Read the model definition and answer for the solid it produces. Units are mm, in the model's axes. A direction names the side the tool comes from. Coordinates: 2 decimals unless noted, no trailing zeros. Write each loop counter-clockwise with the first axis right and the second up, starting at its lowest first coordinate (ties: lowest second). Pieces come first, ordered by that corner, then holes. Notation, with made-up numbers: (20.5, 56) - (74.5, 56) arc R29 ccw to (74.5, 78) - close; hole circle Ø10 at (-2.75, 3). An arc over 180 degrees is marked (long way). Use a Markdown table: item, result.
from build123d import *

# Parameters (mm, degrees)
F1_DEPTH = 3.175
F2_R     = 1.27


with BuildPart() as f1:
    # F0 (on Top) → F1 (new body)
    with BuildSketch(Plane.XY):
        with BuildLine():
            Line((-21.930882, 13.368339), (-2.54, -2.842578))
            Line((-2.54, -2.842578), (-2.54, -18.3762))
            Line((-2.54, -18.3762), (-2.54, -24.069088))
            Line((-2.54, -24.069088), (2.54, -24.069088))
            Line((2.54, -24.069088), (6.35, -24.069088))
            Line((6.35, -24.069088), (6.35, -18.3762))
            Line((6.35, -18.3762), (2.54, -18.3762))
            Line((2.54, -18.3762), (2.54, -2.842578))
            Line((2.54, -2.842578), (21.930882, 13.368339))
            ThreePointArc((21.930882, 13.368339), (23.67951, 37.005537), (0, 38.032972))
            ThreePointArc((0, 38.032972), (-23.67951, 37.005537), (-21.930882, 13.368339))
        make_face()
        with BuildLine():
            Line((19.48717, 16.291415), (0, 0))
            Line((0, 0), (-19.48717, 16.291415))
            ThreePointArc((-19.48717, 16.291415), (-19.234192, 35.984614), (0, 31.75))
            ThreePointArc((0, 31.75), (19.234192, 35.984614), (19.48717, 16.291415))
        make_face(mode=Mode.SUBTRACT)
    extrude(amount=F1_DEPTH)

    # F2
    f2_edges = [f1.edges().sort_by_distance(p)[0] for p in [
        (-12.235441, 5.262881, 3.175),
        (-23.67951, 37.005537, 3.175),
        (23.67951, 37.005537, 3.175),
        (12.235441, 5.262881, 3.175),
        (-2.54, -13.455833, 3.175),
        (2.54, -10.609389, 3.175),
        (-9.743585, 8.145707, 0),
        (-19.234192, 35.984614, 3.175),
        (19.234192, 35.984614, 3.175),
        (4.445, -18.3762, 3.175),
        (6.35, -21.222644, 3.175),
        (1.905, -24.069088, 3.175),
    ]]
    fillet(f2_edges, radius=F2_R)


solid = f1.part
(1) For faces 4 (the flat face through (-9.607, 8.032, 1.583)), 5 (the flat face through (6.35, -21, 1)), 6 (the cylindrical face through (-9.71, 7.65, 2.79)), 7 (the flat face through (4, -18.376, 1)), 8 (the cylindrical face through (11.914, 5.467, 2.793)), determine the directions among +Z, -Z, +X, -X, +Y, -Y from which every point of the face is accessible in a straight line to the end or side of a thin tool.
Report:
| item | result |
|---|---|
| face 4 | +Z, -Z |
| face 5 | +Z, -Z, +X, -Y |
| face 6 | +Z |
| face 7 | +Z, -Z, +X |
| face 8 | +Z, +X |
(2) The mould has two halves that part along Y. Classify faces 1 (the cylindrical face through (9.426, 7.409, 2.793)), 2 (the cylindrical face through (23.92, 36.73, 0.94)), 3 (the flat face through (-12.4, 5.4, 0.9)): pulls with the +Y half, pulls with the -Y half, needs draft (parallel to the pull), parting line crosses it, or undercut.
Report:
| item | result |
|---|---|
| face 1 | undercut |
| face 2 | parting line crosses it |
| face 3 | pulls with the -Y half |
(3) A cutting plane is placed at B-B, the plane y = -13. Write down the section's boundary in (x, z) (3 decimals), and give its area (3 significant figures).
Report:
| item | result |
|---|---|
| outline | (-2.54, 0) - (2.54, 0) - (2.54, 1.905) arc R1.27 ccw to (1.27, 3.175) - (-1.27, 3.175) arc R1.27 ccw to (-2.54, 1.905) - close |
| area | 15.4 mm² |
(4) A cutting plane is placed at C-C, the plane y = 35. Count the separate pieces of the cut face and the enclosed holes in it, and give its area (3 significant figures).
Report:
| item | result |
|---|---|
| separate pieces | 3 |
| enclosed holes | 0 |
| area | 42.1 mm² |
(5) Straight lines are drawn through the part: L1, parallel to X at y = 36, z = 0.4 (3 decimals); L2, parallel to X at y = -5.5, z = 1.2; L3, parallel to Y at x = 3, z = 0.55. For each, find the intervals that lie inside material, in ascending order.
Report:
| item | result |
|---|---|
| L1 | x = -24.505 to -19.76, -2.923 to 3.468, 19.215 to 24.505 |
| L2 | x = -2.54 to 2.54 |
| L3 | y = -24.07 to -18.38, -2.46 to 2.51, 35.61 to 40.28 |
(6) A cutting plane is placed at A-A, the plane z = 2.65. Write down the section's boundary in (x, y) (3 decimals), and give its area (3 significant figures).
Report:
| item | result |
|---|---|
| outline | (-21.776, 13.554) - (-2.299, -2.73) - (-2.299, -23.828) - (6.109, -23.828) - (6.109, -18.618) - (2.299, -18.618) - (2.299, -2.73) - (21.776, 13.554) arc R16.269 ccw (long way) to (0, 37.698) arc R16.269 ccw (long way) to start; hole (-19.642, 16.106) - (0, -0.315) - (19.642, 16.106) arc R12.941 ccw (long way) to (0, 32.268) arc R12.941 ccw (long way) to start |
| area | 617 mm² |
(7) Each of these flat-tipped pins is pushed along its axis until it touches: P1, Ø1.5, axis at x = 3.5, z = 0.5, coming from the +Y side; P2, Ø1.5, axis at y = -7.5, z = 1, coming from the +X side; P3, Ø0.6, axis at y = -22.5, z = 1, coming from the +X side. Where does it stop, or does it pass through?
Report:
| item | result |
|---|---|
| P1 | stops at y = 40.94 |
| P2 | stops at x = 2.54 |
| P3 | stops at x = 6.35 |
